```python
from build123d import *

# Parameters (mm, degrees)
FILLET1_R = 0.5


with BuildPart() as part:
    # Sketch3 → Revolve2 (revolve)
    with BuildSketch(Plane(origin=(0, 0, 0), x_dir=(1, 0, 0), z_dir=(0, 1, 0)), mode=Mode.PRIVATE) as revolve2_sk:
        Polygon((8, 0), (8, -35), (5.25, -37.75), (5.25, -40), (5, -40), (5, 0), align=None)
    revolve(revolve2_sk.sketch.rotate(Axis((0, 0, 0), (0, 0, 1)), 180), axis=Axis((0, 0, 0), (0, 0, 1)))

    # Fillet1
    # the kernel refuses this fillet: 0.5 mm, written as the material it adds along each edge
    with BuildSketch(Plane(origin=(0, 0, 37.75), x_dir=(-1, 0, 0), z_dir=(0, 1, 0))) as fillet1_piece_1:
        with BuildLine():
            CenterArc((5.25 + FILLET1_R, FILLET1_R * 0.414213562373), FILLET1_R, 180, 45)
            Line((5.25, FILLET1_R * 0.414213562373), (5.25, 0))
            Line((5.25, 0), (5.25 + FILLET1_R * 0.292893218813, -FILLET1_R * 0.292893218813))
        make_face()
    revolve(axis=Axis((0, 0, 37.75), (0, 0, 1)))
    # the kernel refuses this fillet: 0.5 mm, written as the material it takes off along each edge
    with BuildSketch(Plane(origin=(0, 0, 0), x_dir=(-1, 0, 0), z_dir=(0, 1, 0))) as fillet1_2_piece_1:
        with BuildLine():
            CenterArc((8 - FILLET1_R, FILLET1_R), FILLET1_R, 270, 90)
            Line((8 - FILLET1_R, 0), (8, 0))
            Line((8, 0), (8, FILLET1_R))
        make_face()
    revolve(axis=Axis((0, 0, 0), (0, 0, 1)), mode=Mode.SUBTRACT)
    with BuildSketch(Plane(origin=(0, 0, 35), x_dir=(-1, 0, 0), z_dir=(0, 1, 0))) as fillet1_2_piece_2:
        with BuildLine():
            CenterArc((8 - FILLET1_R, -FILLET1_R * 0.414213562373), FILLET1_R, 0, 45)
            Line((8 - FILLET1_R * 0.292893218813, FILLET1_R * 0.292893218813), (8, 0))
            Line((8, 0), (8, -FILLET1_R * 0.414213562373))
        make_face()
    revolve(axis=Axis((0, 0, 35), (0, 0, 1)), mode=Mode.SUBTRACT)
    with BuildSketch(Plane(origin=(0, 0, 40), x_dir=(-1, 0, 0), z_dir=(0, 1, 0))) as fillet1_2_piece_3:
        with BuildLine():
            CenterArc((4.75, -0.433012702), FILLET1_R, 0, 60)
            Line((5.25, -0.433012702), (5.25, 0))
            Line((5.25, 0), (5, 0))
        make_face()
    revolve(axis=Axis((0, 0, 40), (0, 0, 1)), mode=Mode.SUBTRACT)
    with BuildSketch(Plane(origin=(0, 0, 0), x_dir=(-1, 0, 0), z_dir=(0, 1, 0))) as fillet1_2_piece_4:
        with BuildLine():
            CenterArc((5 + FILLET1_R, FILLET1_R), FILLET1_R, 180, 90)
            Line((5, FILLET1_R), (5, 0))
            Line((5, 0), (5 + FILLET1_R, 0))
        make_face()
    revolve(axis=Axis((0, 0, 0), (0, 0, 1)), mode=Mode.SUBTRACT)


solid = part.part
```
Could you check a few things on this model? Use its own coordinates, in mm. A direction names the side the tool comes from. Coordinates: 2 decimals unless noted, no trailing zeros. Write each loop counter-clockwise with the first axis right and the second up, starting at its lowest first coordinate (ties: lowest second). Pieces come first, ordered by that corner, then holes. Notation, with made-up numbers: (0, 78.5) -> (56, 78.5) arc R29 cw to (56, 105.5) -> close; hole circle Ø5 at (45.25, 35). An arc over 180 degrees is marked (long way). Return JSON: item names as keys, results as strings.
(1) Imagine slicing it at A-A, the plane y = 0. Please give me the cut outline in (x, z), then the cut area to 3 significant figures.
Numbers:
{"outline": "(-8, 0.5) arc R0.5 ccw to (-7.5, 0) -> (-5.5, 0) arc R0.5 ccw to (-5, 0.5) -> (-5, 40) arc R0.5 ccw to (-5.25, 39.57) -> (-5.25, 37.96) arc R0.5 cw to (-5.4, 37.6) -> (-7.85, 35.15) arc R0.5 ccw to (-8, 34.79) -> close; (5, 0.5) arc R0.5 ccw to (5.5, 0) -> (7.5, 0) arc R0.5 ccw to (8, 0.5) -> (8, 34.79) arc R0.5 ccw to (7.85, 35.15) -> (5.4, 37.6) arc R0.5 cw to (5.25, 37.96) -> (5.25, 39.57) arc R0.5 ccw to (5, 40) -> close", "area": "220 mm2"}
(2) Which directions (+Z, -Z, +X, -X, +Y, -Y) give clear straight access to the entire face, cutting with the end or side of a thin tool? Please do faces 4 (the cylindrical face through (-5, -1.6, 38.8)), 5 (the cylindrical face through (1.73, 7.81, 17.89)).
Numbers:
{"face 4": "+Z", "face 5": "+Z, -Z"}
(3) I'm going to push flat-ended pins straight in: pin 1 (1 mm diameter, centred on y = 4, z = 6.5, fed in from -X); pin 2 (6 mm diameter, centred on x = 0, y = 0, fed in from -Z) (3 decimals); pin 3 (5 mm diameter, centred on y = 5, z = 21, fed in from +X). Where does each tip first touch, or does it pass through?
Numbers:
{"pin 1": "stops at x = -7.19", "pin 2": "passes through", "pin 3": "stops at x = 7.6"}
(4) I need wall thicknesses on L1, parallel to X at y = 0, z = 10.5; L2, parallel to X at y = -3.25, z = 29. Which ranges of each line are inside material? Lowest first, please.
Numbers:
{"L1": "x = -8 to -5, 5 to 8", "L2": "x = -7.31 to -3.8, 3.8 to 7.31"}
(5) Imagine slicing it at D-D, the plane z = 36. Please give me the cut outline in (x, y).
Numbers:
{"outline": "circle Ø14 at (0, 0); hole circle Ø10 at (0, 0)"}
(6) We'd pull the mould along Y, two halves only. Please class faces 1 (the flat face through (-4, -4, 0)), 2 (the conical face through (-2.545, 4.893, 37.484)), 3 (the cylindrical face through (5, 0, 20)): +Y half, -Y half, draft (parallel to the pull), parting line (faces both ways), or undercut.
Numbers:
{"face 1": "draft", "face 2": "parting line", "face 3": "undercut"}
(7) Imagine slicing it at C-C, the plane z = 7.5. Please give me the cut outline in (x, y).
Numbers:
{"outline": "circle Ø16 at (0, 0); hole circle Ø10 at (0, 0)"}
